from build123d import *

# Parameters (mm, degrees)
F0_R     = 3.175
F1_DEPTH = 3.048


with BuildPart() as f1:
    # F0 (on Front) → F1 (new body)
    with BuildSketch(Plane.XZ):
        with BuildLine():
            ThreePointArc((0, 59.5809938932), (-3.9190061068, 63.5), (0, 67.4190061068))
            Line((0, 67.4190061068), (0, 79.375))
            ThreePointArc((0, 79.375), (-10.5003255158, 75.40625), (-15.7504882737, 65.484375))
            Line((-15.7504882737, 65.484375), (-15.7504882737, 61.515625))
            ThreePointArc((-15.7504882737, 61.515625), (-10.5003255158, 51.59375), (0, 47.625))
            Line((0, 47.625), (0, 59.5809938932))
        make_face()
        with BuildLine():
            Line((0, 79.375), (0, 67.4190061068))
            ThreePointArc((0, 67.4190061068), (2.7711557936, 66.2711557936), (3.9190061068, 63.5))
            ThreePointArc((3.9190061068, 63.5), (2.7711557936, 60.7288442064), (0, 59.5809938932))
            Line((0, 59.5809938932), (0, 47.625))
            ThreePointArc((0, 47.625), (10.7468179803, 51.8157572647), (15.8196447136, 62.1754373797))
            ThreePointArc((15.8196447136, 62.1754373797), (15.8611551412, 62.8371405988), (15.875, 63.5))
            ThreePointArc((15.875, 63.5), (15.8438414904, 64.4941387366), (15.7504882737, 65.484375))
            ThreePointArc((15.7504882737, 65.484375), (10.5003255158, 75.40625), (0, 79.375))
        make_face()
        with BuildLine():
            ThreePointArc((-15.7504882737, 65.484375), (-10.5003255158, 75.40625), (0, 79.375))
            Line((0, 79.375), (0, 100.0252))
            Line((0, 100.0252), (0, 104.775))
            ThreePointArc((0, 104.775), (-7.14375, 107.9998046905), (-9.4502929642, 115.490625))
            Line((-9.4502929642, 115.490625), (-15.7504882737, 65.484375))
        make_face()
        with Locations((-3.175, 100.0252)):
            Circle(F0_R, mode=Mode.SUBTRACT)
        with BuildLine():
            Line((0, 100.0252), (0, 79.375))
            ThreePointArc((0, 79.375), (10.5003255158, 75.40625), (15.7504882737, 65.484375))
            Line((15.7504882737, 65.484375), (9.4502929642, 115.490625))
            ThreePointArc((9.4502929642, 115.490625), (9.5063048942, 114.896483242), (9.525, 114.3))
            ThreePointArc((9.525, 114.3), (6.7351920908, 107.5648079092), (0, 104.775))
            Line((0, 104.775), (0, 100.0252))
        make_face()
        with BuildLine():
            Line((0, 10.5767495189), (0, 47.625))
            ThreePointArc((0, 47.625), (-10.5003255158, 51.59375), (-15.7504882737, 61.515625))
            Line((-15.7504882737, 61.515625), (-8.7490265409, 5.9432453232))
            ThreePointArc((-8.7490265409, 5.9432453232), (-4.9501218809, 9.3468670553), (0, 10.5767495189))
        make_face()
        with BuildLine():
            ThreePointArc((15.8196447136, 62.1754373797), (10.7468179803, 51.8157572647), (0, 47.625))
            Line((0, 47.625), (0, 10.5767495189))
            ThreePointArc((0, 10.5767495189), (7.4788913077, 7.4788913077), (10.5767495189, 0))
            Line((10.5767495189, 0), (24.9921450567, 0))
            ThreePointArc((24.9921450567, 0), (27.5436570711, 5.8305265344), (33.5578243434, 7.9126036823))
            Line((33.5578243434, 7.9126036823), (19.3829058745, 9.037946304))
            ThreePointArc((19.3829058745, 9.037946304), (13.9520765692, 11.8171520245), (12.0896121754, 17.6265511124))
            Line((12.0896121754, 17.6265511124), (15.8196447136, 62.1754373797))
        make_face()
        with BuildLine():
            Line((-15.7504882737, 61.515625), (-15.7504882737, 65.484375))
            ThreePointArc((-15.7504882737, 65.484375), (-15.875, 63.5), (-15.7504882737, 61.515625))
        make_face()
        with BuildLine():
            ThreePointArc((10.5767495189, 0), (7.4788913077, 7.4788913077), (0, 10.5767495189))
            ThreePointArc((0, 10.5767495189), (-4.9501218809, 9.3468670553), (-8.7490265409, 5.9432453232))
            ThreePointArc((-8.7490265409, 5.9432453232), (-9.3468670553, -4.9501218809), (0, -10.5767495189))
            Line((0, -10.5767495189), (1.6688517724, -10.4442598659))
            ThreePointArc((1.6688517724, -10.4442598659), (8.0473181112, -6.8635487616), (10.5767495189, 0))
        make_face()
        with BuildLine():
            ThreePointArc((4.322937818, 0), (-3.0567786457, -3.0567786457), (0, 4.322937818))
            ThreePointArc((0, 4.322937818), (3.0567786457, 3.0567786457), (4.322937818, 0))
        make_face(mode=Mode.SUBTRACT)
        with BuildLine():
            ThreePointArc((-9.4502929642, 115.490625), (-7.14375, 107.9998046905), (0, 104.775))
            ThreePointArc((0, 104.775), (6.7351920908, 107.5648079092), (9.525, 114.3))
            ThreePointArc((9.525, 114.3), (9.5063048942, 114.896483242), (9.4502929642, 115.490625))
            ThreePointArc((9.4502929642, 115.490625), (0, 123.825), (-9.4502929642, 115.490625))
        make_face()
        with BuildLine():
            ThreePointArc((3.175, 114.3), (2.2450640303, 112.0549359697), (0, 111.125))
            ThreePointArc((0, 111.125), (-2.2450640303, 116.5450640303), (3.175, 114.3))
        make_face(mode=Mode.SUBTRACT)
        with BuildLine():
            Line((24.9921450567, 0), (10.5767495189, 0))
            ThreePointArc((10.5767495189, 0), (8.0473181112, -6.8635487616), (1.6688517724, -10.4442598659))
            Line((1.6688517724, -10.4442598659), (33.5578243434, -7.9126036823))
            ThreePointArc((33.5578243434, -7.9126036823), (27.5436570711, -5.8305265344), (24.9921450567, 0))
        make_face()
        with BuildLine():
            Line((1.6688517724, -10.4442598659), (0, -10.5767495189))
            ThreePointArc((0, -10.5767495189), (0.8370513345, -10.5435750791), (1.6688517724, -10.4442598659))
        make_face()
        with BuildLine():
            ThreePointArc((33.5578243434, 7.9126036823), (27.5436570711, 5.8305265344), (24.9921450567, 0))
            ThreePointArc((24.9921450567, 0), (27.5436570711, -5.8305265344), (33.5578243434, -7.9126036823))
            ThreePointArc((33.5578243434, -7.9126036823), (38.7601715912, -5.3859879856), (40.8671450567, 0))
            ThreePointArc((40.8671450567, 0), (38.7601715912, 5.3859879856), (33.5578243434, 7.9126036823))
        make_face()
        with BuildLine():
            ThreePointArc((36.4792131905, 0), (32.9296450567, -3.5495681337), (29.380076923, 0))
            ThreePointArc((29.380076923, 0), (32.9296450567, 3.5495681337), (36.4792131905, 0))
        make_face(mode=Mode.SUBTRACT)
    extrude(amount=F1_DEPTH)


solid = f1.part
Could you check a few things on this model? Use its own coordinates, in mm. A direction names the side the tool comes from. Give positions to 0.01 mm unless a question says otherwise; leave off trailing zeros. Loops run counter-clockwise (first coordinate to the right, second up) from the corner with the lowest first, then second, coordinate; pieces in that order, holes last. Notation, with made-up numbers: (1, 29) -> (44, 29) arc R16 cw to (44, 39) -> close; hole circle Ø4 at (66.5, 80). An arc over 180 degrees is marked (long way). Answer as CSV lines item,"result". Start each with the question number.
(1) Which directions (+Z, -Z, +X, -X, +Y, -Y) give clear straight access to the entire face, cutting with the end or side of a thin tool? Please do faces 5 (the flat face through (13.93, -1.5, 39.59)), 6 (the flat face through (-12.3, -1.5, 34.12)), 7 (the flat face through (26.57, -1.503, 8.467)).
(2) I need wall thicknesses on probe 1 along Z at (x, y) = (2.5, -0.4); probe 2 along X at (y, z) = (-1.5, 2); probe 3 along Z at (x, y) = (-0.5, -1.3). Which ranges of each line are inside material? Lowest first, please.
(3) I'm going to push flat-ended pins straight in: pin 1 Ø1 at (x, y) = (32, -2.5) entering from +Z; pin 2 Ø1 at (x, y) = (24.5, -1) entering from +Z. Where does each tip first touch, or does it pass through?
(4) If we section it at C-C on z = 107.5: Write out the boundary of the cut face in (x, y).
(5) If we section it at B-B on x = 27: Write out the boundary of the cut face in (y, z), then the cut area to 3 significant figures.
(6) We'd pull the mould along Z, two halves only. Please class faces 1 (the flat face through (6, 0, 58)), 2 (the cylindrical face through (-15.875, -1.503, 63.528)), 3 (the cylindrical face through (-3.588, -1.503, 103.173)), 4 (the flat face through (17.39, -1.503, -9.196)): released by +Z, released by -Z, zero draft, split by the parting line, or undercut.
(7) If we section it at A-A on y = -1.6: Count the separate pieces of the cut face and the enclosed holes in it, then the cut area to 3 significant figures.
Computed:
1,face 5,"+X, +Y, -Y"
1,face 6,"-X, +Y, -Y"
1,face 7,"+Z, +X, +Y, -Y"
2,probe 1,"z = -10.38 to -3.53, 3.53 to 60.48, 66.52 to 112.34, 116.26 to 123.49"
2,probe 2,"x = -10.39 to -3.83, 3.83 to 30, 35.86 to 40.61"
2,probe 3,"z = -10.56 to -4.29, 4.29 to 59.61, 67.39 to 98.31, 101.74 to 111.16, 117.44 to 123.81"
3,pin 1,"stops at z = 8.08"
3,pin 2,"stops at z = 8.67"
4,outline,"(-10.46, -3.05) -> (10.46, -3.05) -> (10.46, 0) -> (-10.46, 0) -> close"
5,outline,"(-3.05, -8.43) -> (0, -8.43) -> (0, 8.43) -> (-3.05, 8.43) -> close"
5,area,"51.4 mm2"
6,face 1,"zero draft"
6,face 2,"split by the parting line"
6,face 3,"undercut"
6,face 4,"released by -Z"
7,separate pieces,"1"
7,enclosed holes,"5"
7,area,"3,550 mm2"
